The figure shows three views and two pictorial views of one solid part (mm, origin at its lowest corner). Answer the questions. Round coordinates to 2 decimals unless told otherwise and drop trailing zeros. Write each loop counter-clockwise with the first axis right and the second up, starting at its lowest first coordinate (ties: lowest second). Pieces come first, ordered by that corner, then holes. Notation, with made-up numbers: M -38.75,-21.5 L 0.25,-21.5 A15 ccw 0.25,-5.5 Z; hole C 73,-15.5 d7. An arc over 180 degrees is marked long. Answer in a Markdown table with one row per item.
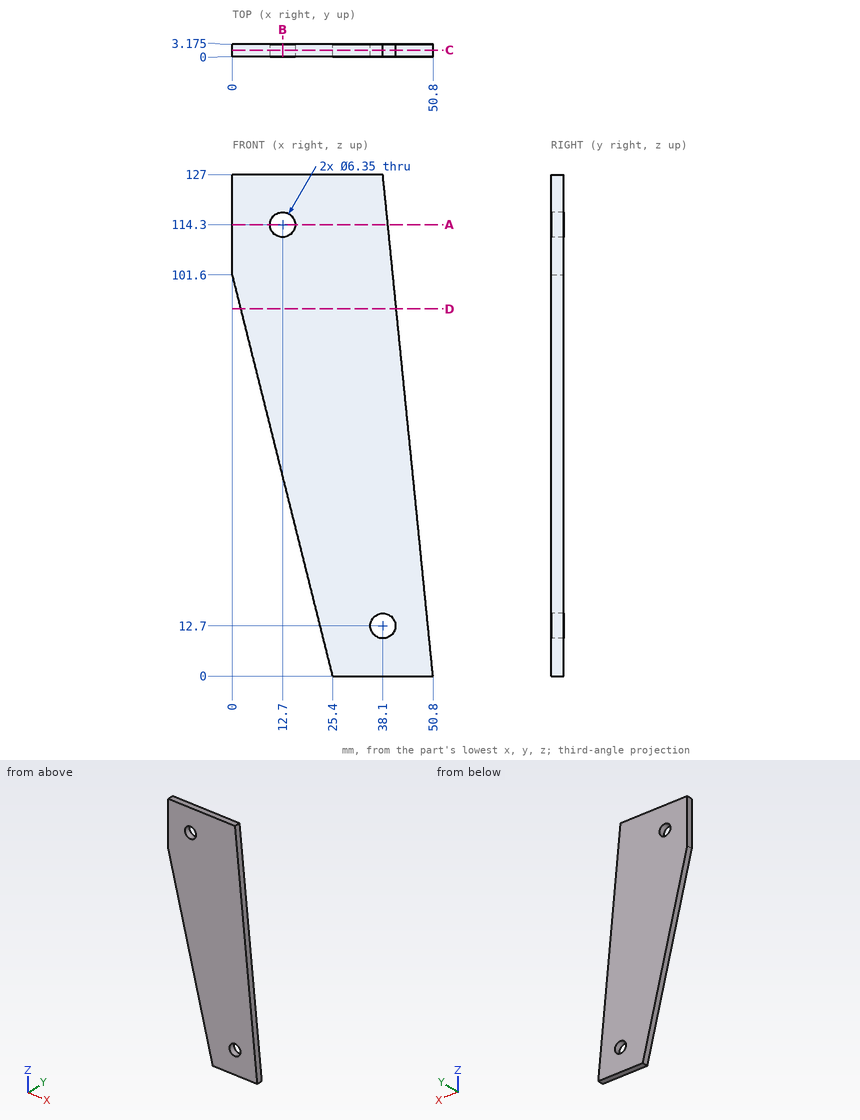
1. Consider line 1 along X through (y, z) = (1.75, 13.5) (3 decimals); line 2 along Z through (x, y) = (36.5, 0.9); line 3 along X through (y, z) = (2.05, 5). Determine where each line is inside the solid, lowest interval first. Write a range as from..to.
Calculated:
| item | result |
|---|---|
| line 1 | x = 22.025..35.027, 41.173..49.45 |
| line 2 | z = 0..9.96, 15.44..127 |
| line 3 | x = 24.15..50.3 |
2. The part is cut by section A-A (z = 114.3). Determine the outline of the cut face in (x, y) (3 decimals), plus the area to 3 significant figures.
Calculated:
| item | result |
|---|---|
| outline | M 0,0 L 9.525,0 L 9.525,3.175 L 0,3.175 Z; M 15.875,0 L 39.37,0 L 39.37,3.175 L 15.875,3.175 Z |
| area | 105 mm² |
3. The part is cut by section D-D (z = 93). Determine the outline of the cut face in (x, y) (3 decimals), plus the area to 3 significant figures.
Calculated:
| item | result |
|---|---|
| outline | M 2.15,0 L 41.5,0 L 41.5,3.175 L 2.15,3.175 Z |
| area | 125 mm² |
4. The part is cut by section B-B (x = 12.7). Determine the outline of the cut face in (y, z) (3 decimals).
Calculated:
| item | result |
|---|---|
| outline | M 0,50.8 L 3.175,50.8 L 3.175,111.125 L 0,111.125 Z; M 0,117.475 L 3.175,117.475 L 3.175,127 L 0,127 Z |
5. The part is cut by section C-C (y = 1.65). Determine the outline of the cut face in (x, z) (3 decimals), plus the area to 3 significant figures.
Calculated:
| item | result |
|---|---|
| outline | M 0,101.6 L 25.4,0 L 50.8,0 L 38.1,127 L 0,127 Z; hole C 12.7,114.3 d6.35; hole C 38.1,12.7 d6.35 |
| area | 4,290 mm² |
